Part model, mm, in its own coordinate system. Coordinates: 2 decimals unless noted, no trailing zeros. Write each loop counter-clockwise with the first axis right and the second up, starting at its lowest first coordinate (ties: lowest second). Pieces come first, ordered by that corner, then holes. Notation, with made-up numbers: (61.25, -29) - (116.25, -29) arc R20 ccw to (116.25, -20) - close; hole circle Ø5 at (79, 35.25). An arc over 180 degrees is marked (long way). Use a Markdown table: item, result.
```python
from build123d import *

# Parameters (mm, degrees)
EXTRUDE_1_DEPTH = 40
EXTRUDE_2_DEPTH = 40


with BuildPart() as part:
    # 草图1 → 凸台-拉伸1 (new body)
    with BuildSketch(Plane.XY):
        Polygon((-115, 0), (115, 0), (115, -5), (-115.278668015, -5), (-322.519573187, 18.17254404), (-511.63276316, 59.025714898), (-681.043594869, 111.694020512), (-830.167599932, 170.615996068), (-959.898827689, 231.441774436), (-1079.263175746, 295.015855057), (-1180.937012969, 355.121645311), (-1178.392557068, 359.425799603), (-1076.814515779, 299.376640342), (-957.66086644, 235.914778968), (-828.185710586, 175.209062462), (-679.380389192, 116.413005408), (-510.360191041, 63.866144258), (-321.711807872, 23.113383276), align=None)
    extrude_1 = extrude(amount=EXTRUDE_1_DEPTH)

    # 草图2 → 凸台-拉伸2 (add)
    with BuildSketch(Plane.XY.offset(40)):
        Polygon((-115, 0), (-113.88877965, 9.938067686), (-115.876393187, 10.160311756), (-116.987613537, 0.22224407), align=None)
        Polygon((-321.711807872, 23.113383276), (-320.600587522, 33.051450962), (-318.612973985, 32.829206892), (-319.724194334, 22.891139206), align=None)
        Polygon((-510.360191041, 63.866144258), (-508.248649021, 73.640671883), (-506.293743496, 73.21836348), (-508.405285516, 63.443835854), align=None)
        Polygon((-679.380389192, 116.413005408), (-676.411639975, 125.962169146), (-674.501807228, 125.368419302), (-677.470556445, 115.819255565), align=None)
        Polygon((-828.185710586, 175.209062462), (-824.51095702, 184.509395049), (-822.650890502, 183.774444336), (-826.325644068, 174.474111749), align=None)
        Polygon((-957.66086644, 235.914778968), (-953.41571144, 244.968985671), (-951.604870099, 244.119954671), (-955.850025099, 235.065747968), align=None)
        Polygon((-1076.814515779, 299.376640342), (-1072.113637159, 308.20283659), (-1070.34839791, 307.262660865), (-1075.04927653, 298.436464618), align=None)
        Polygon((-1178.392557068, 359.425799603), (-1173.303645267, 368.034108187), (-1171.58198355, 367.016325826), (-1176.670895352, 358.408017242), align=None)
    extrude_2 = extrude(amount=-EXTRUDE_2_DEPTH)

    # 镜向1: 凸台-拉伸1, 凸台-拉伸2 across plane
    add(extrude_1.mirror(Plane(origin=(0, 0, 0), x_dir=(0, 0, 1), z_dir=(1, 0, 0))))
    add(extrude_2.mirror(Plane(origin=(0, 0, 0), x_dir=(0, 0, 1), z_dir=(1, 0, 0))))


solid = part.part
```
Item 1: Band-saw the part on B-B, the plane x = -53.5. Give the cut face in (y, z).
From the geometry:
| item | result |
|---|---|
| outline | (-5, 0) - (0, 0) - (0, 40) - (-5, 40) - close |
Item 2: Drill centre lines: probe 1 along X at (y, z) = (342.5, 21.5); probe 2 along X at (y, z) = (248, 11); probe 3 along Y at (x, z) = (-567, 19.5). Where is each one in solid material? Low to high.
From the geometry:
| item | result |
|---|---|
| probe 1 | -1159.59 to -1149.76, 1149.76 to 1159.59 |
| probe 2 | -990.99 to -980.35, 980.35 to 990.99 |
| probe 3 | 76.24 to 81.47 |
Item 3: Drop flat-ended pins along their axis: P1, Ø12, axis at x = -443.5, z = 7, coming from the +Y side; P2, Ø3, axis at y = 293.5, z = 17.5, coming from the +X side; P3, Ø4, axis at y = 277, z = 25, coming from the -X side. Give the stop position or say it passes through.
From the geometry:
| item | result |
|---|---|
| P1 | y = 50.72 |
| P2 | x = 1079.23 |
| P3 | x = -1049.19 |
Item 4: Two-plate mould, pull along X, no slides. Class faces 1 (the face through (1129.39, 324.65, 19.72)), 2 (the face through (-894.125, 200.603, 19.72)), 3 (the face through (1127.442, 329.306, 19.72)), 4 (the face through (2, -5, 20)): pulls with the +X half, pulls with the -X half, needs draft (parallel to the pull), parting line crosses it, or undercut.
From the geometry:
| item | result |
|---|---|
| face 1 | pulls with the +X half |
| face 2 | pulls with the -X half |
| face 3 | undercut |
| face 4 | needs draft |
Item 5: Band-saw the part on C-C, the plane x = -648.5. Give the cut face in (y, z).
From the geometry:
| item | result |
|---|---|
| outline | (101.58, 0) - (106.81, 0) - (106.81, 40) - (101.58, 40) - close |
Item 6: Band-saw the part on A-A, the plane y = 333.5. Give the cut face in (x, z), then the cut area to 3 significant figures.
From the geometry:
| item | result |
|---|---|
| outline | (-1144.36, 0) - (-1134.54, 0) - (-1134.54, 40) - (-1144.36, 40) - close; (1134.54, 0) - (1144.36, 0) - (1144.36, 40) - (1134.54, 40) - close |
| area | 786 mm^2 |
